Autodesk Inventor part; units mm, degrees
ref_plane "YZ Plane" through (0, 0, 0) normal (1, 0, 0) x (0, 1, 0)
ref_plane "XZ Plane" through (0, 0, 0) normal (0, 1, 0) x (-1, 0, 0)
ref_plane "XY Plane" through (0, 0, 0) normal (0, 0, 1) x (1, 0, 0)
sketch "スケッチ1" plane through (0, 0, 0) normal (0, 0, 1) x (1, 0, 0)
  circle A0 centre (0, 0) radius 2
  dimension "d0" = 4
extrude "押し出し1" add sketch "スケッチ1" along normal blind 6
sketch "スケッチ2" plane through (0, 0, 6) normal (0, 0, 1) x (1, 0, 0)
  circle A0 centre (0, 0) radius 2
  circle A1 centre (0, 0) radius 4
  dimension "d3" = 8
extrude "押し出し2" add sketch "スケッチ2" along normal blind 2.3 contours A0 | A1
thread "ねじ1"
chamfer "面取り1" distance 2 angle 45 1 edges at (-4, 0, 6)
sketch "スケッチ4" plane through (0, 0, 0) normal (0, 0, -1) x (-1, 0, 0)
  circle A0 centre (0, 0) radius 2
extrude "押し出し4" add sketch "スケッチ4" along normal blind 11.7
properties part number "SB　M4 20mm 皿ネジ" material "Stainless Steel, 440C"
Verification items for the finished model (mm, model axes). Give positions to 0.01 mm unless a question says otherwise; leave off trailing zeros. Order: outer loops, then holes, each group sorted by start corner. A loop starts at its lowest first (then second) coordinate and runs counter-clockwise, first axis right, second up. Notation, with made-up numbers: M -8,-30 L 10,-30 A22 ccw 10,0 Z; hole C 79,20.25 d6. An arc over 180 degrees is marked long. Return JSON: item names as keys, results as strings. Group by question number.
1) Scan lines: line 1 (X direction, y = 0, z = -1.5); line 2 (Z direction, x = -0.5, y = 3); line 3 (Z direction, x = 1, y = -2.25). Record each from-to range of solid material in increasing order.
2) Go/stop test with flat-tipped pins: pin 1 Ø1.5 at (y, z) = (-3, -0.5) entering from -X; pin 2 Ø2 at (x, z) = (-1.5, -3.5) entering from -Y; pin 3 Ø1 at (x, y) = (-2, -0.5) entering from -Z; pin 4 Ø1 at (y, z) = (-0.5, 3.5) entering from +X. Record where each tip stops, or that it passes through.
3) Section check C-C on z = -7.25. Record the cut outline in (x, y), and give its area (3 significant figures).
Answer block:
{
 "1": {"line 1": "x = -2 to 2", "line 2": "z = 7.04 to 8.3", "line 3": "z = 6.46 to 8.3"},
 "2": {"pin 1": "passes through", "pin 2": "stops at y = -1.94", "pin 3": "stops at z = -11.7", "pin 4": "stops at x = 2"},
 "3": {"outline": "C 0,0 d4", "area": "12.6 mm^2"}
}
